from build123d import *

# Parameters (mm, degrees)
CUT_EXTRUDE1_DEPTH = 17
SKETCH3_W          = 12
SKETCH3_H          = 16
CHAMFER1_SIZE2     = 1.000000021
CHAMFER1_SIZE      = 1.000000018
CHAMFER2_SIZE      = 0.5
SCALE1_SCALE       = 0.75


with BuildPart() as part:
    # Sketch1 → Revolve1 (revolve)
    with BuildSketch(Plane(origin=(0, 0, 0), x_dir=(1, 0, 0), z_dir=(0, 1, 0))):
        Polygon((43, 8), (0, 8), (0, -8), (43, -8), (43, -6.003672577), (32, -2), (32, 2), (43, 6.003672577), align=None)
    revolve(axis=Axis((0, 0, -8), (0, 0, 1)))

    # Sketch2 → Cut-Extrude1 (cut, through all)
    with BuildSketch(Plane.XY.offset(8)):
        with BuildLine():
            Line((-15, -4), (-11.313708499, -4))
            ThreePointArc((-11.313708499, -4), (-12, -1e-09), (-11.313708499, 3.999999999))
            Line((-11.313708499, 3.999999999), (-15, 3.999999999))
            Line((-15, 3.999999999), (-15, -4))
        make_face()
    extrude(amount=-CUT_EXTRUDE1_DEPTH, mode=Mode.SUBTRACT)

    # Sketch3 → Cut-Revolve1 (revolve, cut)
    with BuildSketch(Plane(origin=(0, 0, 0), x_dir=(1, 0, 0), z_dir=(0, 1, 0))):
        with Locations((6, 0)):
            Rectangle(SKETCH3_W, SKETCH3_H)
    revolve(axis=Axis((0, 0, -8), (0, 0, 1)), mode=Mode.SUBTRACT)

    # Chamfer1
    chamfer1_edges = [part.edges().sort_by_distance(p)[0] for p in [
        (12, 1e-09, -8),
        (12, 1e-09, 8),
    ]]
    chamfer(chamfer1_edges, length=CHAMFER1_SIZE, length2=CHAMFER1_SIZE2)

    # Chamfer2
    chamfer2_edges = [part.edges().sort_by_distance(p)[0] for p in [
        (-43, 0, 8),
        (-43, 0, -8),
    ]]
    chamfer(chamfer2_edges, length=CHAMFER2_SIZE)


with BuildPart() as part_1:
    # Scale1: scaled about (0.084922045, 0, 0)
    add(part.part.scale(SCALE1_SCALE).moved(Location((0.021230511, 0, 0))))


solid = part_1.part
Can you work these out from the model? Positions are in its coordinate system, mm. A direction names the side the tool comes from. Round coordinates to 2 decimals unless told otherwise and drop trailing zeros. Loops run counter-clockwise (first coordinate to the right, second up) from the corner with the lowest first, then second, coordinate; pieces in that order, holes last. Notation, with made-up numbers: (72.5, 7.25) - (105.5, 7.25) arc R26 cw to (105.5, 43.25) - close; hole circle Ø4 at (83.25, 6). An arc over 180 degrees is marked (long way). Use CSV: the item, a comma, the result in double quotes. Start each with the question number.
1) We'd pull the mould along Y, two halves only. Please class faces 1 (the flat face through (-10, 3, 0)), 2 (the flat face through (-10, -3, 0)), 3 (the conical face through (-5.268, -23.82, 1.646)), 4 (the flat face through (7, 8, -6)): released by +Y, released by -Y, zero draft, split by the parting line, or undercut.
2) If we section it at B-B on z = 3.75: Write out the boundary of the cut face in (x, y), plus the area to 3 significant figures.
3) Please list where these lines run through material, in increasing order: probe 1 along Y at (x, z) = (-0.5, -0.75); probe 2 along Z at (x, y) = (23.5, 14); probe 3 along Z at (x, y) = (25.5, 4.5). Write a range as [from, to].
4) If we section it at A-A on y = 0: Write out the boundary of the cut face in (x, z) (3 decimals).
5) For faces 5 (the flat face through (-11.229, 0, 0)), 6 (the conical face through (23.41, 7.36, -1.69)), 7 (the flat face through (-7, 8, 6)), which set-ups out of +Z, -Z, +X, -X, +Y, -Y let a thin tool reach every point of the face, with its end or its side?
6) For pin 1 Ø3 at (x, z) = (-9.5, -4) entering from -Y, with a flat end and sliding along its axis, tell me the tip position at first contact or that it passes through.
Geometry results:
1,face 1,"undercut"
1,face 2,"undercut"
1,face 3,"split by the parting line"
1,face 4,"zero draft"
2,outline,"circle Ø60.36 at (0.02, 0); hole (-11.23, -3) - (-8.46, -3) arc R9 ccw (long way) to (-8.46, 3) - (-11.23, 3) - close"
2,area,"2,590 mm2"
3,probe 1,"y = [-23.99, -8.98], [8.98, 23.99]"
3,probe 2,"z = [-6, -2.71], [2.71, 6]"
3,probe 3,"z = [-6, -2.18], [2.18, 6]"
4,outline,"(-32.229, -5.625) - (-31.854, -6) - (-11.229, -6) - (-11.229, 6) - (-31.854, 6) - (-32.229, 5.625) - (-32.229, 4.503) - (-23.979, 1.5) - (-23.979, -1.5) - (-32.229, -4.503) - close; (9.021, -5.25) - (9.771, -6) - (31.896, -6) - (32.271, -5.625) - (32.271, -4.503) - (24.021, -1.5) - (24.021, 1.5) - (32.271, 4.503) - (32.271, 5.625) - (31.896, 6) - (9.771, 6) - (9.021, 5.25) - close"
5,face 5,"+Z, -Z"
5,face 6,"none"
5,face 7,"+Z, +X, -X, +Y, -Y"
6,pin 1,"stops at y = -31.21"
